Check sheet for the drawn part. Datum: minimum x, y, z corner. Units: mm. A direction names the side the tool comes from. Coordinates: 2 decimals unless noted, no trailing zeros. Order: outer loops, then holes, each group sorted by start corner. A loop starts at its lowest first (then second) coordinate and runs counter-clockwise, first axis right, second up.
1. Draft check along Z on the marked faces 3, 4 and 5. Enter one of: released by +Z, released by -Z, zero draft, split by the parting line, or undercut.
2. Set-up check for the marked faces 1 and 2: record each of +Z, -Z, +X, -X, +Y, -Y from which the full face is reachable in a straight line by a thin tool's end or side.
3. Gauge pin test, flat ends, axial feed: pin 1 Ø15 at (x, z) = (89, 14) entering from +Y; pin 2 Ø1 at (y, z) = (25.5, 29) entering from +X. Record the tip position at first contact, or that the pin passes through.
4. Thickness scan on line 1 (Y direction, x = 60, z = 7.5); line 2 (Y direction, x = 10, z = 4.5). Record the ranges inside material, lowest first.
5. Cross-section at A-A (z = 21). Enter the section's corners in (x, y).
6. Cross-section at B-B (y = 55). Enter the section's corners in (x, z), then the cut area to 3 significant figures.
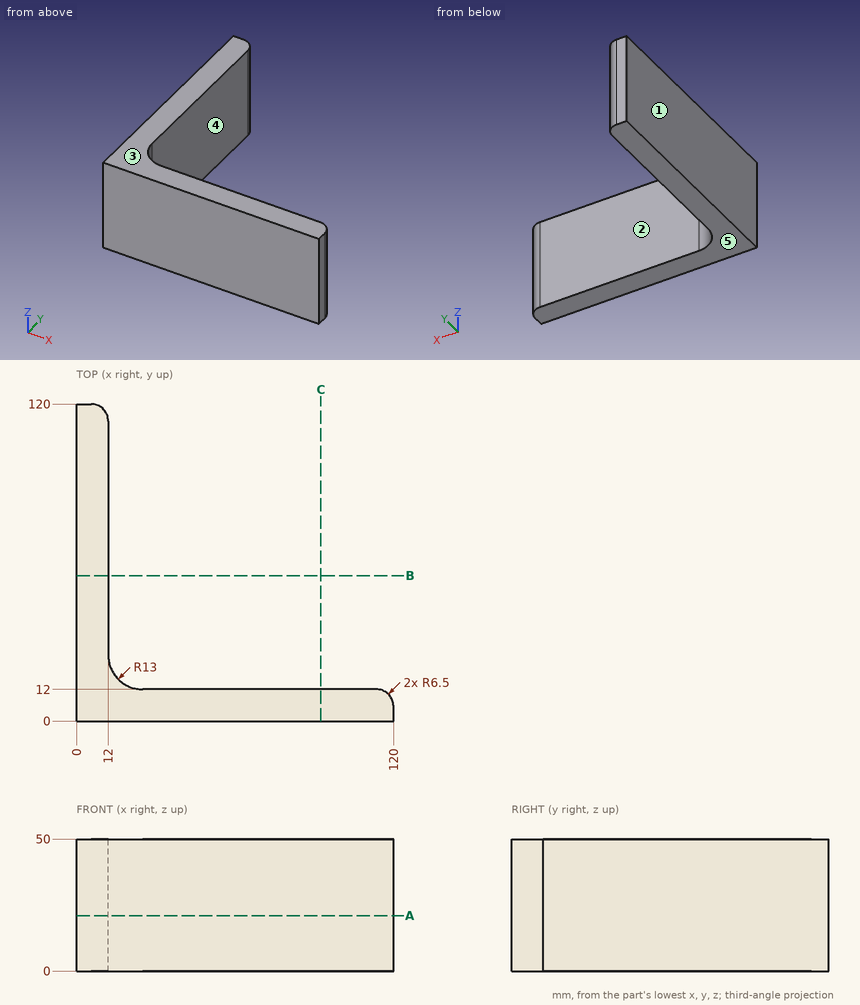
Data:
1. face 3: released by +Z
1. face 4: zero draft
1. face 5: released by -Z
2. face 1: +Z, -Z, -X, +Y, -Y
2. face 2: +Z, -Z, +X, +Y
3. pin 1: stops at y = 12
3. pin 2: stops at x = 12
4. line 1: y = 0 to 12
4. line 2: y = 0 to 118.19
5. outline: (0, 0) - (120, 0) - (120, 5.5) arc R6.5 ccw to (113.5, 12) - (25, 12) arc R13 cw to (12, 25) - (12, 113.5) arc R6.5 ccw to (5.5, 120) - (0, 120) - close
6. outline: (0, 0) - (12, 0) - (12, 50) - (0, 50) - close
6. area: 600 mm2
